Design review of the part built by this model. Coordinates are the model's own, in mm. Coordinates: 2 decimals unless noted, no trailing zeros. Order: outer loops, then holes, each group sorted by start corner. A loop starts at its lowest first (then second) coordinate and runs counter-clockwise, first axis right, second up. Notation, with made-up numbers: (16.25, 85) -> (34.25, 85) arc R25 ccw to (34.25, 111) -> close; hole circle Ø11 at (-18.5, 64). An arc over 180 degrees is marked (long way). Write item = value, one per line.
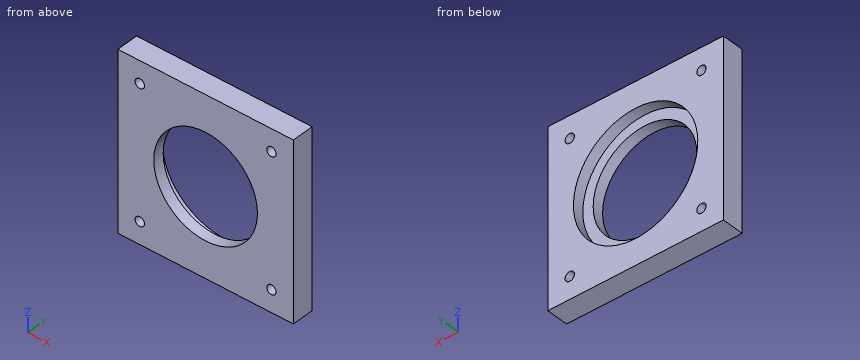
```python
from build123d import *

# Parameters (mm, degrees)
SKETCH2_W                 = 50.8
SKETCH2_H                 = 50.8
BOSS_EXTRUDE1_DEPTH       = 6.35
SKETCH3_R                 = 18
CUT_EXTRUDE1_DEPTH        = 3.175
SKETCH4_R                 = 15
CUT_EXTRUDE2_DEPTH        = 73.122135992
TAP_DRILL_FOR_6_32_TAP1_D = 2.7051


with BuildPart() as part:
    # Sketch2 → Boss-Extrude1 (new body)
    with BuildSketch(Plane(origin=(0, 0, 0), x_dir=(1, 0, 0), z_dir=(0, 1, 0))):
        with Locations((-25.4, 25.4)):
            Rectangle(SKETCH2_W, SKETCH2_H)
    extrude(amount=BOSS_EXTRUDE1_DEPTH)

    # Sketch3 → Cut-Extrude1 (cut)
    with BuildSketch(Plane(origin=(0, 6.35, 0), x_dir=(1, 0, 0), z_dir=(0, 1, 0))):
        with Locations(Location((-25.4, 25.4, 0), (0, 0, 270))):
            Circle(SKETCH3_R)
    extrude(amount=-CUT_EXTRUDE1_DEPTH, mode=Mode.SUBTRACT)

    # Sketch4 → Cut-Extrude2 (cut, through all)
    with BuildSketch(Plane(origin=(0, 0, 0), x_dir=(-1, 0, 0), z_dir=(0, -1, 0))):
        with Locations(Location((25.4, 25.4, 0), (0, 0, 90))):
            Circle(SKETCH4_R)
    extrude(amount=-CUT_EXTRUDE2_DEPTH, mode=Mode.SUBTRACT)

    # Tap Drill for #6-32 Tap1 (through all)
    with Locations(Plane(origin=(0, 0, 0), x_dir=(-1, 0, 0), z_dir=(0, -1, 0))):
        with Locations((6.35, 6.35), (6.35, 44.45), (44.45, 44.45), (44.45, 6.35), (25.4, 25.4)):
            Hole(TAP_DRILL_FOR_6_32_TAP1_D / 2)


solid = part.part
```
(1) We need section C-C (y = 2.5). Write out the cut boundary in (x, z).
Report:
outline = (-50.8, -50.8) -> (0, -50.8) -> (0, 0) -> (-50.8, 0) -> close; hole circle Ø2.71 at (-44.45, -44.45); hole circle Ø2.71 at (-44.45, -6.35); hole circle Ø30 at (-25.4, -25.4); hole circle Ø2.71 at (-6.35, -44.45); hole circle Ø2.71 at (-6.35, -6.35)
(2) We need section A-A (z = -6.35). Write out the cut boundary in (x, y).
Report:
outline = (-50.8, 0) -> (-45.8, 0) -> (-45.8, 6.35) -> (-50.8, 6.35) -> close; (-43.1, 0) -> (-7.7, 0) -> (-7.7, 6.35) -> (-43.1, 6.35) -> close; (-5, 0) -> (0, 0) -> (0, 6.35) -> (-5, 6.35) -> close
(3) For L1, parallel to Z at x = -6.5, y = 3.5; L2, parallel to X at y = 3.75, z = -44.45; L3, parallel to X at y = 0.95, z = -25.4, list the stretches that pass through material, from the lowest coordinate up.
Report:
L1 = -50.8 to -45.79, -43.11 to -7.69, -5.01 to 0
L2 = -50.8 to -45.8, -43.1 to -7.7, -5 to 0
L3 = -50.8 to -40.4, -10.4 to 0
(4) We need section D-D (z = -25.4). Write out the cut boundary in (x, y) (3 decimals).
Report:
outline = (-50.8, 0) -> (-40.4, 0) -> (-40.4, 3.175) -> (-43.4, 3.175) -> (-43.4, 6.35) -> (-50.8, 6.35) -> close; (-10.4, 0) -> (0, 0) -> (0, 6.35) -> (-7.4, 6.35) -> (-7.4, 3.175) -> (-10.4, 3.175) -> close
(5) We need section B-B (x = -44.45). Write out the cut boundary in (y, z).
Report:
outline = (0, -50.8) -> (6.35, -50.8) -> (6.35, -45.8) -> (0, -45.8) -> close; (0, -43.1) -> (6.35, -43.1) -> (6.35, -7.7) -> (0, -7.7) -> close; (0, -5) -> (6.35, -5) -> (6.35, 0) -> (0, 0) -> close
(6) Insertion check: pin 1 (1 mm diameter, centred on x = -16, z = -11.5, fed in from +Y) (3 decimals). The pin has a flat end and moves straight along its axis. Give the tip position at first contact, or say it passes through.
Report:
pin_1 = 3.175
